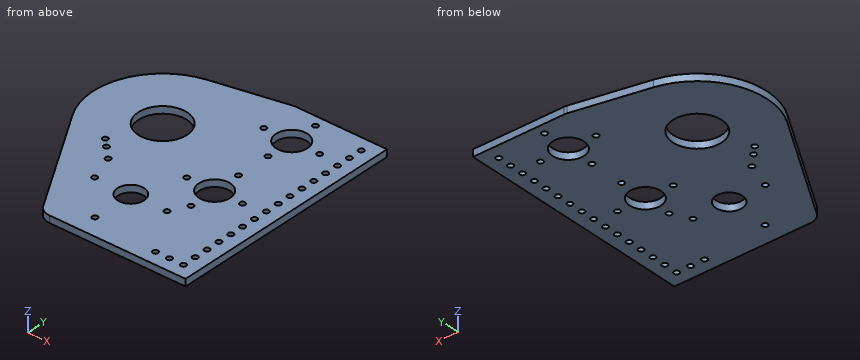
from build123d import *

# Parameters (mm, degrees)
SKETCH1_R                          = 22.225
SKETCH1_R_2                        = 14.2875
SKETCH1_R_3                        = 12.065
BOSS_EXTRUDE1_DEPTH                = 6.35
F_9_0_196_DIAMETER_HOLE1_OUTLINE_R = 2.4892
F_9_0_196_DIAMETER_HOLE1_DEPTH     = 6.35
SKETCH5_W                          = 158.475738421
SKETCH5_H                          = 23.945509926
CUT_EXTRUDE1_DEPTH                 = 198.577920905
FILLET1_R                          = 12.7


# Read off the part's stored shape, not the designer's step: #9 (0.196) Diameter Hole1
with BuildPart() as part:
    # Sketch1 → Boss-Extrude1 (new body)
    with BuildSketch(Plane(origin=(0, 0, 0), x_dir=(0, 1, 0), z_dir=(0, 0, 1))):
        with BuildLine():
            Line((80.9625, -82.55), (80.9625, -139.7))
            Line((80.9625, -139.7), (-139.573, -139.7))
            Line((-139.573, -139.7), (-139.573, -8.2804))
            Line((-139.573, -8.2804), (-32.138994776, 54.766184957))
            ThreePointArc((-32.138994776, 54.766184957), (25.818013961, 58.014482288), (62.200093141, 12.782738878))
            Line((62.200093141, 12.782738878), (80.150058213, -74.560788201))
            ThreePointArc((80.150058213, -74.560788201), (80.758867143, -78.534792445), (80.9625, -82.55))
        make_face()
        with Locations(Location((0, 0, 0), (0, 0, 270))):
            Circle(SKETCH1_R, mode=Mode.SUBTRACT)
        with Locations(Location((-41.275, -82.55, 0), (0, 0, 270))):
            Circle(SKETCH1_R_2, mode=Mode.SUBTRACT)
        with Locations(Location((41.275, -82.55, 0), (0, 0, 270))):
            Circle(SKETCH1_R_2, mode=Mode.SUBTRACT)
        with Locations(Location((-82.55, -41.275, 0), (0, 0, 270))):
            Circle(SKETCH1_R_3, mode=Mode.SUBTRACT)
    extrude(amount=BOSS_EXTRUDE1_DEPTH)

    # #9 (0.196) Diameter Hole1 outline → #9 (0.196) Diameter Hole1 (cut)
    with BuildSketch(Plane.XY):
        with Locations((101.6, -127)):
            Circle(F_9_0_196_DIAMETER_HOLE1_OUTLINE_R)
        with Locations((114.3, -127)):
            Circle(F_9_0_196_DIAMETER_HOLE1_OUTLINE_R)
        with Locations((127, 63.5)):
            Circle(F_9_0_196_DIAMETER_HOLE1_OUTLINE_R)
        with Locations((127, 50.8)):
            Circle(F_9_0_196_DIAMETER_HOLE1_OUTLINE_R)
        with Locations((127, 38.1)):
            Circle(F_9_0_196_DIAMETER_HOLE1_OUTLINE_R)
        with Locations((127, 25.4)):
            Circle(F_9_0_196_DIAMETER_HOLE1_OUTLINE_R)
        with Locations((127, 12.7)):
            Circle(F_9_0_196_DIAMETER_HOLE1_OUTLINE_R)
        with Locations((127, 0)):
            Circle(F_9_0_196_DIAMETER_HOLE1_OUTLINE_R)
        with Locations((8.2804, -82.55)):
            Circle(F_9_0_196_DIAMETER_HOLE1_OUTLINE_R)
        with Locations((41.275, -121.031)):
            Circle(F_9_0_196_DIAMETER_HOLE1_OUTLINE_R)
        with Locations((74.2696, -82.55)):
            Circle(F_9_0_196_DIAMETER_HOLE1_OUTLINE_R)
        with Locations((0, -58.355558977)):
            Circle(F_9_0_196_DIAMETER_HOLE1_OUTLINE_R)
        with Locations((-10.779281546, -47.582226654)):
            Circle(F_9_0_196_DIAMETER_HOLE1_OUTLINE_R)
        with Locations((-17.965469244, -40.400005105)):
            Circle(F_9_0_196_DIAMETER_HOLE1_OUTLINE_R)
        with Locations((127, -12.7)):
            Circle(F_9_0_196_DIAMETER_HOLE1_OUTLINE_R)
        with Locations((127, -25.4)):
            Circle(F_9_0_196_DIAMETER_HOLE1_OUTLINE_R)
        with Locations((127, -38.1)):
            Circle(F_9_0_196_DIAMETER_HOLE1_OUTLINE_R)
        with Locations((127, -50.8)):
            Circle(F_9_0_196_DIAMETER_HOLE1_OUTLINE_R)
        with Locations((127, -63.5)):
            Circle(F_9_0_196_DIAMETER_HOLE1_OUTLINE_R)
        with Locations((127, -76.2)):
            Circle(F_9_0_196_DIAMETER_HOLE1_OUTLINE_R)
        with Locations((127, -88.9)):
            Circle(F_9_0_196_DIAMETER_HOLE1_OUTLINE_R)
        with Locations((127, -101.6)):
            Circle(F_9_0_196_DIAMETER_HOLE1_OUTLINE_R)
        with Locations((127, -114.3)):
            Circle(F_9_0_196_DIAMETER_HOLE1_OUTLINE_R)
        with Locations((127, -127)):
            Circle(F_9_0_196_DIAMETER_HOLE1_OUTLINE_R)
        with Locations((107.95, -41.275)):
            Circle(F_9_0_196_DIAMETER_HOLE1_OUTLINE_R)
        with Locations((82.55, -66.675)):
            Circle(F_9_0_196_DIAMETER_HOLE1_OUTLINE_R)
        with Locations((57.15, -41.275)):
            Circle(F_9_0_196_DIAMETER_HOLE1_OUTLINE_R)
        with Locations((82.55, -15.875)):
            Circle(F_9_0_196_DIAMETER_HOLE1_OUTLINE_R)
        with Locations((82.55, 15.875)):
            Circle(F_9_0_196_DIAMETER_HOLE1_OUTLINE_R)
        with Locations((107.95, 41.275)):
            Circle(F_9_0_196_DIAMETER_HOLE1_OUTLINE_R)
        with Locations((82.55, 66.675)):
            Circle(F_9_0_196_DIAMETER_HOLE1_OUTLINE_R)
        with Locations((57.15, 41.275)):
            Circle(F_9_0_196_DIAMETER_HOLE1_OUTLINE_R)
    extrude(amount=F_9_0_196_DIAMETER_HOLE1_DEPTH, mode=Mode.SUBTRACT)

    # Sketch5 → Cut-Extrude1 (cut, through all)
    with BuildSketch(Plane.XY.offset(6.35)):
        with Locations((102.364485766, 88.172754963)):
            Rectangle(SKETCH5_W, SKETCH5_H)
    extrude(amount=-CUT_EXTRUDE1_DEPTH, mode=Mode.SUBTRACT)

    # Fillet1
    fillet1_edges = [part.edges().sort_by_distance(p)[0] for p in [
        (8.2804, -139.573, 3.175),
        (55.340025647, 76.2, 3.175),
    ]]
    fillet(fillet1_edges, radius=FILLET1_R)


solid = part.part
Check sheet for the modelled part. Datum: model origin and axes. Units: mm. Coordinates: 2 decimals unless noted, no trailing zeros. Loops run counter-clockwise (first coordinate to the right, second up) from the corner with the lowest first, then second, coordinate; pieces in that order, holes last. Notation, with made-up numbers: (-2, 34) -> (35, 34) arc R13 cw to (35, 43) -> close; hole circle Ø5 at (16.5, -2). An arc over 180 degrees is marked (long way). Write item = value, one per line. Start each with the question number.
1. Section check A-A on x = 114.3. Record the cut outline in (y, z).
2. Section check B-B on y = -82.55. Record the cut outline in (x, z).
3. Material ranges on line 1 (Y direction, x = 57.15, z = 2.25); line 2 (Y direction, x = 40, z = 1.5); line 3 (Y direction, x = 114, z = 2.75), recorded low to high.
4. Section check C-C on z = 3. Give the number of separate pieces and of enclosed holes in the cut face, then the cut area to 3 significant figures.
5. Depth check by flat-ended pin: P1, Ø6.5, axis at x = 82.55, y = -66.675, coming from the -Z side; P2, Ø1.5, axis at y = -18.5, z = 3.5, coming from the -X side; P3, Ø3, axis at y = -112, z = 4.5, coming from the -X side. Enter the tip coordinate at first touch or a pass-through.
Responses:
q1.outline = (-139.57, 0) -> (-129.49, 0) -> (-129.49, 6.35) -> (-139.57, 6.35) -> close; (-124.51, 0) -> (76.2, 0) -> (76.2, 6.35) -> (-124.51, 6.35) -> close
q2.outline = (-25.18, 0) -> (5.79, 0) -> (5.79, 6.35) -> (-25.18, 6.35) -> close; (10.77, 0) -> (29.21, 0) -> (29.21, 6.35) -> (10.77, 6.35) -> close; (53.34, 0) -> (71.78, 0) -> (71.78, 6.35) -> (53.34, 6.35) -> close; (76.76, 0) -> (139.7, 0) -> (139.7, 6.35) -> (76.76, 6.35) -> close
q3.line_1 = -139.57 to -43.76, -38.79 to 38.79, 43.76 to 76.2
q3.line_2 = -139.57 to -123.17, -118.89 to -94.55, -70.55 to 73.05
q3.line_3 = -139.57 to -129.47, -124.53 to 76.2
q4.separate_pieces = 1
q4.enclosed_holes = 36
q4.area = 33,500 mm2
q5.P1 = 0
q5.P2 = -60.97
q5.P3 = -8.78
